from build123d import *

# Parameters (mm, degrees)
F0_R     = 3
F1_DEPTH = 10
F0_R_2   = 4
F2_DEPTH = 4
F3_R     = 2


with BuildPart() as f1:
    # F0 (on Front) → F1 (new body)
    with BuildSketch(Plane.XZ):
        Circle(F0_R)
    extrude(amount=F1_DEPTH)

    # F0 (on Front) → F2 (join)
    with BuildSketch(Plane.XZ):
        Circle(F0_R_2)
        Circle(F0_R, mode=Mode.SUBTRACT)
        Circle(F0_R)
    extrude(amount=-F2_DEPTH)

    # F3
    f3_edges = [f1.edges().sort_by_distance(p)[0] for p in [
        (-4, 4, 0),
    ]]
    fillet(f3_edges, radius=F3_R)


solid = f1.part
The model under review builds one solid part; all positions refer to its coordinate system, in mm. A direction names the side the tool comes from. Coordinates: 2 decimals unless noted, no trailing zeros. Loops run counter-clockwise (first coordinate to the right, second up) from the corner with the lowest first, then second, coordinate; pieces in that order, holes last.
(1) Consider section A-A, the plane y = 1.5. Give the boundary of the cut face in (x, z), plus the area to 3 significant figures.
Determined:
outline: circle Ø8 at (0, 0)
area: 50.3 mm2
(2) Insertion check: P1, Ø2, axis at x = -3, z = 3, coming from the +Y side; P2, Ø1.5, axis at x = -1.5, z = -3, coming from the +Y side. Each pin has a flat end and moves straight along its axis. Give the tip position at first contact, or say it passes through.
Determined:
P1: stops at y = 3.57
P2: stops at y = 3.91
(3) Tool access review of faces 1 (the flat face through (0, 4, 0)), 2 (the cylindrical face through (-3, -5, 0)): name each direction out of +Z, -Z, +X, -X, +Y, -Y from which nothing blocks a thin tool from reaching the whole face with its end or side.
Determined:
face 1: +Z, -Z, +X, -X, +Y
face 2: -Y
(4) Wall thickness on L1, parallel to X at y = 0.25, z = -1.5; L2, parallel to Z at x = 0.75, y = 1.5; L3, parallel to Z at x = 1.25, y = -5.75: over which ranges is each line inside the solid? List them lowest first.
Determined:
L1: x = -3.71 to 3.71
L2: z = -3.93 to 3.93
L3: z = -2.73 to 2.73
